Read the model definition and answer for the solid it produces. Units are mm, in the model's axes. Face numbers are marked on the shaded views. A direction names the side the tool comes from. Coordinates: 2 decimals unless noted, no trailing zeros.
Q1. Flat-ended cylindrical pins translate along their axes: P1, Ø1.8, axis at y = 5.5, z = 39, coming from the -X side; P2, Ø6, axis at x = -27.5, y = -0.5, coming from the -Z side; P3, Ø2.5, axis at y = -5, z = 38.5, coming from the -X side. Find the tip coordinate at first contact, or state that the pin passes through.
Q2. The mould has two halves that part along Y. Classify the marked faces 1, 2 and 3: pulls with the +Y half, pulls with the -Y half, needs draft (parallel to the pull), parting line crosses it, or undercut.
Q3. Straight lines are drawn through the part: line 1 (X direction, y = 0.5, z = 28.5); line 2 (Z direction, x = -19.5, y = -33.5); line 3 (Z direction, x = 26.5, y = 14). For each, find the intervals that lie inside material, in ascending order.
Q4. Which of the six approach directions +Z, -Z, +X, -X, +Y, -Y give full straight-line access (tool end or side, diameter ignored) to the marked faces 4 and 5?
Q5. Section A-A (x = -13) is taken. Count the separate pieces of the cut face and the enclosed holes in it, then the cut area to 3 significant figures.
from build123d import *

# Parameters (mm, degrees)
SKETCH_R        = 3.231406
PAD_DEPTH       = 6
SKETCH001_R     = 39.053421
SKETCH001_R_2   = 36.311054
PAD001_DEPTH    = 50
POCKET_DEPTH    = 21
PAD002_DEPTH    = 44
SKETCH005_R     = 4
POCKET001_DEPTH = 8
SKETCH004_R     = 4
POCKET002_DEPTH = 8
SKETCH006_R     = 2
POCKET003_DEPTH = 33.1588870995
SKETCH007_R     = 2
POCKET004_DEPTH = 33.1588870995
POCKET005_DEPTH = 50.001
SKETCH009_R     = 36.442774
POCKET006_DEPTH = 13
SKETCH010_R     = 37.170227
SKETCH010_R_2   = 20.844548
PAD003_DEPTH    = 5
CHAMFER_SIZE    = 2
POCKET007_DEPTH = 5
SKETCH013_W     = 50.953362
SKETCH013_H     = 47.461643
POCKET008_DEPTH = 24.5


with BuildPart() as part:
    # Sketch → Pad (new body)
    with BuildSketch(Plane.XY):
        with BuildLine():
            ThreePointArc((34.394901, -45.939491), (42.558158875, -42.558158875), (45.939491, -34.394901))
            Line((45.939491, 34.394901), (45.939491, -34.394901))
            ThreePointArc((45.939491, 34.394901), (42.558158875, 42.558158875), (34.394901, 45.939491))
            Line((-34.394901, 45.939491), (34.394901, 45.939491))
            ThreePointArc((-34.394901, 45.939491), (-42.558158875, 42.558158875), (-45.939491, 34.394901))
            Line((-45.939491, -34.394901), (-45.939491, 34.394901))
            ThreePointArc((-45.939491, -34.394901), (-42.558158875, -42.558158875), (-34.394901, -45.939491))
            Line((34.394901, -45.939491), (-34.394901, -45.939491))
        make_face()
        with Locations((-34.394901, 34.394901)):
            Circle(SKETCH_R, mode=Mode.SUBTRACT)
        with Locations((34.394901, 34.394901)):
            Circle(SKETCH_R, mode=Mode.SUBTRACT)
        with Locations((-34.394901, -34.394901)):
            Circle(SKETCH_R, mode=Mode.SUBTRACT)
        with Locations((34.394901, -34.394901)):
            Circle(SKETCH_R, mode=Mode.SUBTRACT)
    extrude(amount=PAD_DEPTH)

    # Sketch001 (on Face14 of Pad) → Pad001 (join)
    with BuildSketch(Plane.XY.offset(6)):
        Circle(SKETCH001_R)
        Circle(SKETCH001_R_2, mode=Mode.SUBTRACT)
    extrude(amount=PAD001_DEPTH)

    # Sketch002 (on Face14 of Pad) → Pocket (cut)
    with BuildSketch(Plane.XY.offset(6)):
        with BuildLine():
            ThreePointArc((-21.5988223559, -31.3292084741), (0, -38.0529687512), (21.5988223559, -31.3292084741))
            Line((21.5988223559, -31.3292084741), (22.7946876619, -32.8694723778))
            ThreePointArc((-22.7946613357, -32.8694906348), (1.60187e-05, -40), (22.7946876619, -32.8694723778))
            Line((-21.5988223559, -31.3292084741), (-22.7946613357, -32.8694906348))
        make_face()
    extrude(amount=POCKET_DEPTH, mode=Mode.SUBTRACT)

    # Sketch003 (on Face24 of Pocket) → Pad002 (join)
    with BuildSketch(Plane.XY.offset(6)):
        with BuildLine():
            ThreePointArc((-33.0264474223, -15.3752616453), (0, -36.43), (33.0264474223, -15.3752616453))
            Line((0, -30.775747), (33.0264474223, -15.3752616453))
            Line((-33.0264474223, -15.3752616453), (0, -30.775747))
        make_face()
    extrude(amount=PAD002_DEPTH)

    # Sketch005 (on Face27 of Pad002) → Pocket001 (cut)
    with BuildSketch(Plane(origin=(11.7877949861, -25.2790079252, 0), x_dir=(-0.906307787, -0.4226182617, 0), z_dir=(-0.4226182617, 0.906307787, 0))):
        with Locations((2, 17)):
            Circle(SKETCH005_R)
    extrude(amount=-POCKET001_DEPTH, mode=Mode.SUBTRACT)

    # Sketch004 (on Face25 of Pad002) → Pocket002 (cut)
    with BuildSketch(Plane(origin=(-11.7877949861, -25.2790079252, 0), x_dir=(-0.906307787, 0.4226182617, 0), z_dir=(0.4226182617, 0.906307787, 0))):
        with Locations((-2, 17)):
            Circle(SKETCH004_R)
    extrude(amount=-POCKET002_DEPTH, mode=Mode.SUBTRACT)

    # Sketch006 (on Face27 of Pad002) → Pocket003 (cut, through all)
    with BuildSketch(Plane(origin=(11.7877949861, -25.2790079252, 0), x_dir=(-0.906307787, -0.4226182617, 0), z_dir=(-0.4226182617, 0.906307787, 0))):
        with Locations((2, 17)):
            Circle(SKETCH006_R)
    extrude(amount=-POCKET003_DEPTH, mode=Mode.SUBTRACT)

    # Sketch007 (on Face25 of Pad002) → Pocket004 (cut, through all)
    with BuildSketch(Plane(origin=(-11.7877949861, -25.2790079252, 0), x_dir=(-0.906307787, 0.4226182617, 0), z_dir=(0.4226182617, 0.906307787, 0))):
        with Locations((-2, 17)):
            Circle(SKETCH007_R)
    extrude(amount=-POCKET004_DEPTH, mode=Mode.SUBTRACT)

    # Sketch008 (on Face28 of Pocket004) → Pocket005 (cut, through all)
    with BuildSketch(Plane.XY.offset(50)):
        with BuildLine():
            ThreePointArc((19.7091874975, -30.8400377462), (0, 36.6), (-19.7091874975, -30.8400377462))
            Line((19.7091874975, -30.8400377462), (-19.7091874975, -30.8400377462))
        make_face()
    extrude(amount=-POCKET005_DEPTH, mode=Mode.SUBTRACT)

    # Sketch009 (on Face20 of Pocket005) → Pocket006 (cut)
    with BuildSketch(Plane.XY.offset(50)):
        Circle(SKETCH009_R)
    extrude(amount=-POCKET006_DEPTH, mode=Mode.SUBTRACT)

    # Sketch010 (on Face21 of Pocket006) → Pad003 (join)
    with BuildSketch(Plane.XY.offset(37)):
        Circle(SKETCH010_R)
        Circle(SKETCH010_R_2, mode=Mode.SUBTRACT)
    extrude(amount=PAD003_DEPTH)

    # Chamfer
    chamfer_edges = [part.edges().sort_by_distance(p)[0] for p in [
        (-20.844548, 0, 42),
    ]]
    chamfer(chamfer_edges, length=CHAMFER_SIZE)

    # Sketch012 (on Face4 of Chamfer) → Pocket007 (cut)
    with BuildSketch(Plane.XY.offset(42)):
        with BuildLine():
            ThreePointArc((-30.5, 3.7080992435), (-33, 0), (-30.5, -3.7080992435))
            Line((-30.5, -3.7080992435), (-30.5, -6))
            ThreePointArc((-30.5, -6), (-29, -7.5), (-27.5, -6))
            Line((-27.5, -6), (-27.5, -3.7080992435))
            ThreePointArc((-27.5, -3.7080992435), (-25, 0), (-27.5, 3.7080992435))
            Line((-27.5, 3.7080992435), (-27.5, 6))
            ThreePointArc((-27.5, 6), (-29, 7.5), (-30.5, 6))
            Line((-30.5, 6), (-30.5, 3.7080992435))
        make_face()
        with BuildLine():
            ThreePointArc((-3.7080992435, 27.5), (0, 25), (3.7080992435, 27.5))
            Line((3.7080992435, 27.5), (6, 27.5))
            ThreePointArc((6, 27.5), (7.5, 29), (6, 30.5))
            Line((6, 30.5), (3.7080992435, 30.5))
            ThreePointArc((3.7080992435, 30.5), (0, 33), (-3.7080992435, 30.5))
            Line((-3.7080992435, 30.5), (-6, 30.5))
            ThreePointArc((-6, 30.5), (-7.5, 29), (-6, 27.5))
            Line((-6, 27.5), (-3.7080992435, 27.5))
        make_face()
        with BuildLine():
            ThreePointArc((27.4981368357, 4.0368241404), (24.9981368357, 0.3287248968), (27.4981368357, -3.3793743467))
            Line((27.4981368357, -3.3793743467), (27.4981368357, -5.6712751032))
            ThreePointArc((27.4981368357, -5.6712751032), (28.9981368357, -7.1712751032), (30.4981368357, -5.6712751032))
            Line((30.4981368357, -5.6712751032), (30.4981368357, -3.3793743467))
            ThreePointArc((30.4981368357, -3.3793743467), (32.9981368357, 0.3287248968), (30.4981368357, 4.0368241404))
            Line((30.4981368357, 4.0368241404), (30.4981368357, 6.3287248968))
            ThreePointArc((30.4981368357, 6.3287248968), (28.9981368357, 7.8287248968), (27.4981368357, 6.3287248968))
            Line((27.4981368357, 6.3287248968), (27.4981368357, 4.0368241404))
        make_face()
    extrude(amount=-POCKET007_DEPTH, mode=Mode.SUBTRACT)

    # Sketch013 (on Face4 of Pocket007) → Pocket008 (cut, symmetric)
    with BuildSketch(Plane.XY.offset(42)):
        with Locations((25.476681, -23.7308215)):
            Rectangle(SKETCH013_W, SKETCH013_H)
    extrude(amount=POCKET008_DEPTH, both=True, mode=Mode.SUBTRACT)


solid = part.part
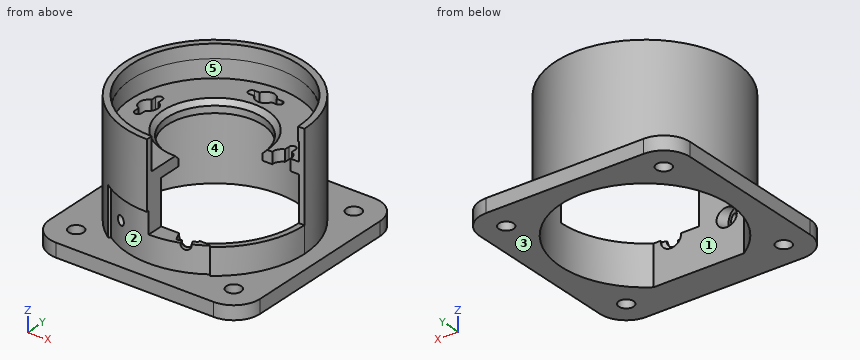
Numbers:
1. P1: stops at x = -38.78
1. P2: stops at z = 37
1. P3: stops at x = -38.87
2. face 1: undercut
2. face 2: pulls with the -Y half
2. face 3: needs draft
3. line 1: x = -39.05 to -36.6, 36.6 to 39.05
3. line 2: z = 0 to 6, 27 to 56
3. line 3: z = 37 to 42
4. face 4: -Z
4. face 5: none
5. separate pieces: 3
5. enclosed holes: 0
5. area: 654 mm2
